For this review, take the finished solid that the model builds, in its own axes (mm). A direction names the side the tool comes from. Round coordinates to 2 decimals unless told otherwise and drop trailing zeros. Order: outer loops, then holes, each group sorted by start corner. A loop starts at its lowest first (then second) coordinate and runs counter-clockwise, first axis right, second up. Notation, with made-up numbers: (58, 24) -> (116, 24) arc R24 ccw to (116, 57) -> close; hole circle Ø11 at (-30.5, 63). An arc over 180 degrees is marked (long way). Answer in a Markdown table with one row per item.
```python
from build123d import *

# Parameters (mm, degrees)
SKETCH1_R           = 1.375
BOSS_EXTRUDE1_DEPTH = 3


with BuildPart() as part:
    # Sketch1 → Boss-Extrude1 (new body)
    with BuildSketch(Plane(origin=(0, 0, 0), x_dir=(1, 0, 0), z_dir=(0, 1, 0))):
        Polygon((12.5, 17.135), (127.2, 17.135), (127.2, 0), (139.7, 0), (139.7, 17.135), (139.7, 27.03449494), (101.68231227, 65.05218267), (38.01768773, 65.05218267), (0, 27.03449494), (0, 17.135), (0, 0), (12.5, 0), align=None)
        with Locations((6.25, 8.5675)):
            Circle(SKETCH1_R, mode=Mode.SUBTRACT)
        with Locations((133.45, 8.5675)):
            Circle(SKETCH1_R, mode=Mode.SUBTRACT)
        with Locations((46.402464035, 27.89462575)):
            Circle(SKETCH1_R, mode=Mode.SUBTRACT)
        with Locations((46.402464035, 42.89462575)):
            Circle(SKETCH1_R, mode=Mode.SUBTRACT)
        with Locations((93.297535965, 27.89462575)):
            Circle(SKETCH1_R, mode=Mode.SUBTRACT)
        with Locations((93.297535965, 42.89462575)):
            Circle(SKETCH1_R, mode=Mode.SUBTRACT)
        with BuildLine():
            Line((55.883073513, 24.04324829), (69.561324865, 33.715232576))
            ThreePointArc((69.561324865, 33.715232576), (69.85, 33.806984285), (70.138675135, 33.715232576))
            Line((70.138675135, 33.715232576), (83.816926487, 24.04324829))
            ThreePointArc((83.816926487, 24.04324829), (84.004761659, 23.483547277), (83.528251352, 23.135))
            Line((83.528251352, 23.135), (56.171748648, 23.135))
            ThreePointArc((56.171748648, 23.135), (55.695238341, 23.483547277), (55.883073513, 24.04324829))
        make_face(mode=Mode.SUBTRACT)
        with BuildLine():
            Line((49.40246404, 27.77516044), (49.40246404, 47.41202223))
            ThreePointArc((49.40246404, 47.41202223), (49.672613618, 47.856059147), (50.191139175, 47.82027052))
            Line((50.191139175, 47.82027052), (64.076497308, 38.001839625))
            ThreePointArc((64.076497308, 38.001839625), (64.287822173, 37.593591335), (64.076497308, 37.185343045))
            Line((64.076497308, 37.185343045), (50.191139175, 27.36691215))
            ThreePointArc((50.191139175, 27.36691215), (49.672613618, 27.331123523), (49.40246404, 27.77516044))
        make_face(mode=Mode.SUBTRACT)
        with BuildLine():
            Line((56.171748648, 52.05218267), (83.528251352, 52.05218267))
            ThreePointArc((83.528251352, 52.05218267), (84.004761659, 51.703635393), (83.816926487, 51.14393438))
            Line((83.816926487, 51.14393438), (70.138675135, 41.471950094))
            ThreePointArc((70.138675135, 41.471950094), (69.85, 41.380198385), (69.561324865, 41.471950094))
            Line((69.561324865, 41.471950094), (55.883073513, 51.14393438))
            ThreePointArc((55.883073513, 51.14393438), (55.695238341, 51.703635393), (56.171748648, 52.05218267))
        make_face(mode=Mode.SUBTRACT)
        with BuildLine():
            Line((90.29753596, 27.77516044), (90.29753596, 47.41202223))
            ThreePointArc((90.29753596, 47.41202223), (90.027386382, 47.856059147), (89.508860825, 47.82027052))
            Line((89.508860825, 47.82027052), (75.623502692, 38.001839625))
            ThreePointArc((75.623502692, 38.001839625), (75.412177827, 37.593591335), (75.623502692, 37.185343045))
            Line((75.623502692, 37.185343045), (89.508860825, 27.36691215))
            ThreePointArc((89.508860825, 27.36691215), (90.027386382, 27.331123523), (90.29753596, 27.77516044))
        make_face(mode=Mode.SUBTRACT)
        with BuildLine():
            Line((15.692388152, 23.135), (40.04777251, 23.135))
            ThreePointArc((40.04777251, 23.135), (40.509712276, 23.443658284), (40.4013259, 23.988553391))
            Line((40.4013259, 23.988553391), (28.223633721, 36.166245569))
            ThreePointArc((28.223633721, 36.166245569), (27.870080331, 36.312692179), (27.51652694, 36.166245569))
            Line((27.51652694, 36.166245569), (15.338834761, 23.988553391))
            ThreePointArc((15.338834761, 23.988553391), (15.230448386, 23.443658284), (15.692388152, 23.135))
        make_face(mode=Mode.SUBTRACT)
        with BuildLine():
            Line((30.344954065, 38.994672694), (42.548910644, 51.198629273))
            ThreePointArc((42.548910644, 51.198629273), (43.093805751, 51.307015649), (43.402464035, 50.845075883))
            Line((43.402464035, 50.845075883), (43.402464035, 26.437162724))
            ThreePointArc((43.402464035, 26.437162724), (43.093805751, 25.975222958), (42.548910644, 26.083609334))
            Line((42.548910644, 26.083609334), (30.344954065, 38.287565913))
            ThreePointArc((30.344954065, 38.287565913), (30.198507456, 38.641119304), (30.344954065, 38.994672694))
        make_face(mode=Mode.SUBTRACT)
        with BuildLine():
            Line((109.355045935, 38.994672694), (97.151089356, 51.198629273))
            ThreePointArc((97.151089356, 51.198629273), (96.606194249, 51.307015649), (96.297535965, 50.845075883))
            Line((96.297535965, 50.845075883), (96.297535965, 26.437162724))
            ThreePointArc((96.297535965, 26.437162724), (96.606194249, 25.975222958), (97.151089356, 26.083609334))
            Line((97.151089356, 26.083609334), (109.355045935, 38.287565913))
            ThreePointArc((109.355045935, 38.287565913), (109.501492544, 38.641119304), (109.355045935, 38.994672694))
        make_face(mode=Mode.SUBTRACT)
        with BuildLine():
            Line((124.361165239, 23.988553391), (112.18347306, 36.166245569))
            ThreePointArc((112.18347306, 36.166245569), (111.829919669, 36.312692179), (111.476366279, 36.166245569))
            Line((111.476366279, 36.166245569), (99.2986741, 23.988553391))
            ThreePointArc((99.2986741, 23.988553391), (99.190287724, 23.443658284), (99.65222749, 23.135))
            Line((99.65222749, 23.135), (124.007611848, 23.135))
            ThreePointArc((124.007611848, 23.135), (124.469551614, 23.443658284), (124.361165239, 23.988553391))
        make_face(mode=Mode.SUBTRACT)
    extrude(amount=BOSS_EXTRUDE1_DEPTH)


solid = part.part
```
Q1. Clearance check with flat-ended pins moving along their axes: pin 1 Ø1.5 at (y, z) = (2.5, -9.5) entering from -X; pin 2 Ø1.5 at (y, z) = (1.5, -34.5) entering from -X; pin 3 Ø1.5 at (y, z) = (2, -43.5) entering from +X; pin 4 Ø0.9 at (y, z) = (1.5, -33) entering from -X. State where each tip first meets the part, or that it passes through.
Answer key:
| item | result |
|---|---|
| pin 1 | stops at x = 0 |
| pin 2 | stops at x = 6.72 |
| pin 3 | stops at x = 123.98 |
| pin 4 | stops at x = 5.52 |
Q2. Take a section at A-A, the plane x = 120. Write out the cut boundary in (y, z) (1 decimal).
Answer key:
| item | result |
|---|---|
| outline | (0, -46.7) -> (3, -46.7) -> (3, -28.3) -> (0, -28.3) -> close; (0, -23.1) -> (3, -23.1) -> (3, -17.1) -> (0, -17.1) -> close |
Q3. To check wall thickness, follow probe 1 along Z at (x, y) = (46.5, 1.4) (3 decimals); probe 2 along Z at (x, y) = (107, 1.5) (1 decimal); probe 3 along X at (y, z) = (2.55, -40). State the ranges of each line that lie inside material, in increasing order.
Answer key:
| item | result |
|---|---|
| probe 1 | z = -65.052 to -44.266, -41.523 to -29.266, -26.523 to -17.135 |
| probe 2 | z = -59.7 to -41.3, -35.9 to -31.7, -23.1 to -17.1 |
| probe 3 | x = 12.97 to 31.35, 43.4 to 49.4, 61.25 to 78.45, 90.3 to 96.3, 108.35 to 126.73 |
Q4. Take a section at B-B, the plane x = 6.25. Write out the cut boundary in (y, z).
Answer key:
| item | result |
|---|---|
| outline | (0, -33.28) -> (3, -33.28) -> (3, -9.94) -> (0, -9.94) -> close; (0, -7.19) -> (3, -7.19) -> (3, 0) -> (0, 0) -> close |
Q5. The part is to be moulded in two halves that separate along Z. For faces 4 (the face through (70, 1, -65.052)), 5 (the face through (70, 1, -23.135)), 6 (the face through (6, 1, 0)), 7 (the face through (12.5, 1, -8)), say which applies: +Z half, -Z half, draft (parallel to the pull), parting line (faces both ways), or undercut.
Answer key:
| item | result |
|---|---|
| face 4 | -Z half |
| face 5 | undercut |
| face 6 | +Z half |
| face 7 | draft |
Q6. Tool access review of faces 1 (the face through (127.2, 1, -9)), 2 (the face through (19.275, 1.479, -46.309)), 3 (the face through (82.663, 1.479, -42.98)): name each direction out of +Z, -Z, +X, -X, +Y, -Y from which nothing blocks a thin tool from reaching the whole face with its end or side.
Answer key:
| item | result |
|---|---|
| face 1 | +Z, +Y, -Y |
| face 2 | -Z, -X, +Y, -Y |
| face 3 | +Y, -Y |
Q7. Take a section at C-C, the plane y = 2.05. Give the number of separate pieces and of enclosed holes in the cut face, then the cut area to 3 significant figures.
Answer key:
| item | result |
|---|---|
| separate pieces | 1 |
| enclosed holes | 14 |
| area | 4,270 mm^2 |
